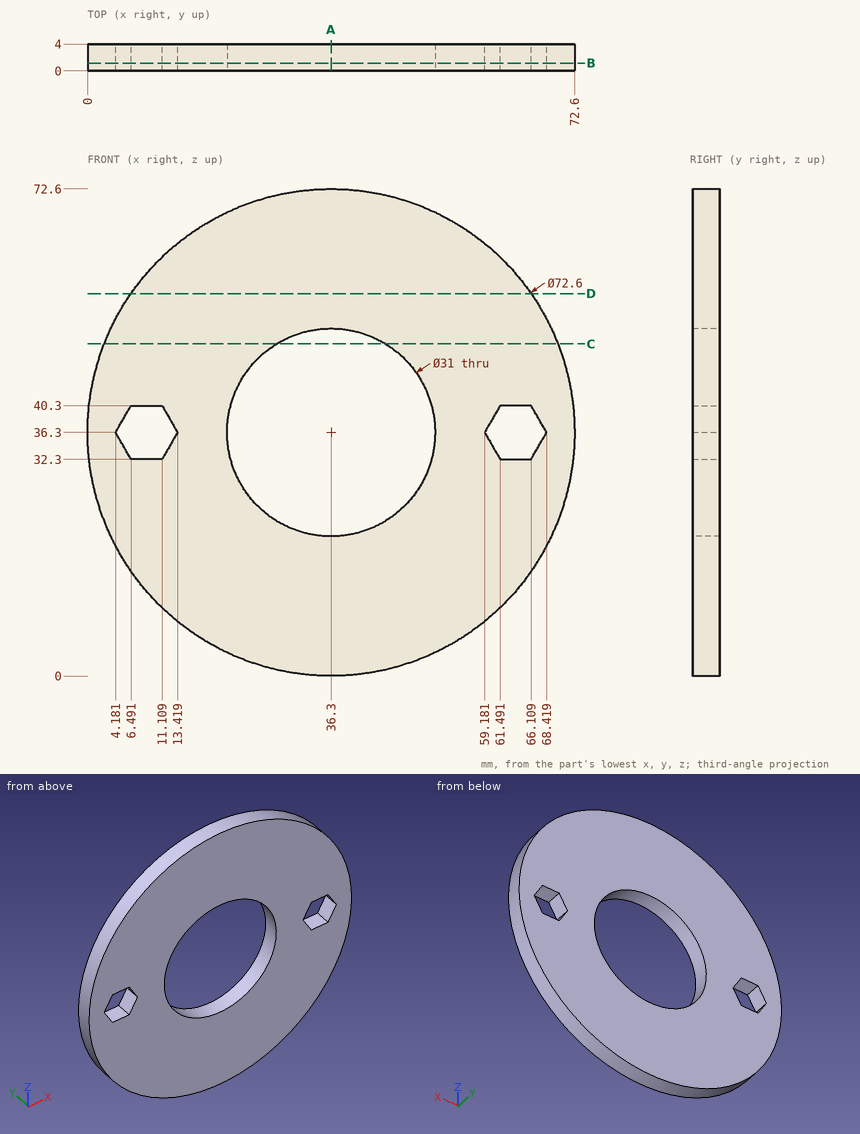
Answer from the drawing. Dimensions are ordinates in mm from the lowest x, y and z of the part. Coordinates: 2 decimals unless noted, no trailing zeros. Loops run counter-clockwise (first coordinate to the right, second up) from the corner with the lowest first, then second, coordinate; pieces in that order, holes last.
1) Section B-B (y = 1.15) is taken. Give the vertices of the cut face in (x, z), plus the area to 3 significant figures.
Results:
outline: circle Ø72.6 at (36.3, 36.3); hole (4.18, 36.3) - (6.49, 32.3) - (11.11, 32.3) - (13.42, 36.3) - (11.11, 40.3) - (6.49, 40.3) - close; hole circle Ø31 at (36.3, 36.3); hole (59.18, 36.3) - (61.49, 32.3) - (66.11, 32.3) - (68.42, 36.3) - (66.11, 40.3) - (61.49, 40.3) - close
area: 3,270 mm2
2) Flat-ended cylindrical pins translate along their axes: pin 1 (2 mm diameter, centred on x = 57, z = 13, fed in from -Y); pin 2 (1.2 mm diameter, centred on x = 64, y = 2.5, fed in from +Z); pin 3 (2 mm diameter, centred on x = 9, y = 3, fed in from -Z); pin 4 (2 mm diameter, centred on x = 64.5, y = 2, fed in from -Z). Find the tip coordinate at first contact, or state that the pin passes through.
Results:
pin 1: stops at y = 0
pin 2: stops at z = 60.45
pin 3: stops at z = 11.28
pin 4: stops at z = 12.26
3) Consider probe 1 along X at (y, z) = (2.6, 36.3); probe 2 along X at (y, z) = (2.2, 39); probe 3 along Z at (x, y) = (62.5, 1.8) (1 decimal). Determine where each line is inside the solid, lowest interval first.
Results:
probe 1: x = 0 to 4.18, 13.42 to 20.8, 51.8 to 59.18, 68.42 to 72.6
probe 2: x = 0.1 to 5.74, 11.86 to 21.04, 51.56 to 60.74, 66.86 to 72.5
probe 3: z = 11.2 to 32.3, 40.3 to 61.4
4) Section A-A (x = 36.3) is taken. Give the vertices of the cut face in (y, z), plus the area to 3 significant figures.
Results:
outline: (0, 0) - (4, 0) - (4, 20.8) - (0, 20.8) - close; (0, 51.8) - (4, 51.8) - (4, 72.6) - (0, 72.6) - close
area: 166 mm2
5) Section D-D (z = 57) is taken. Give the vertices of the cut face in (x, y).
Results:
outline: (6.48, 0) - (66.12, 0) - (66.12, 4) - (6.48, 4) - close
6) Section C-C (z = 49.5) is taken. Give the vertices of the cut face in (x, y) (1 decimal).
Results:
outline: (2.5, 0) - (28.2, 0) - (28.2, 4) - (2.5, 4) - close; (44.4, 0) - (70.1, 0) - (70.1, 4) - (44.4, 4) - close
